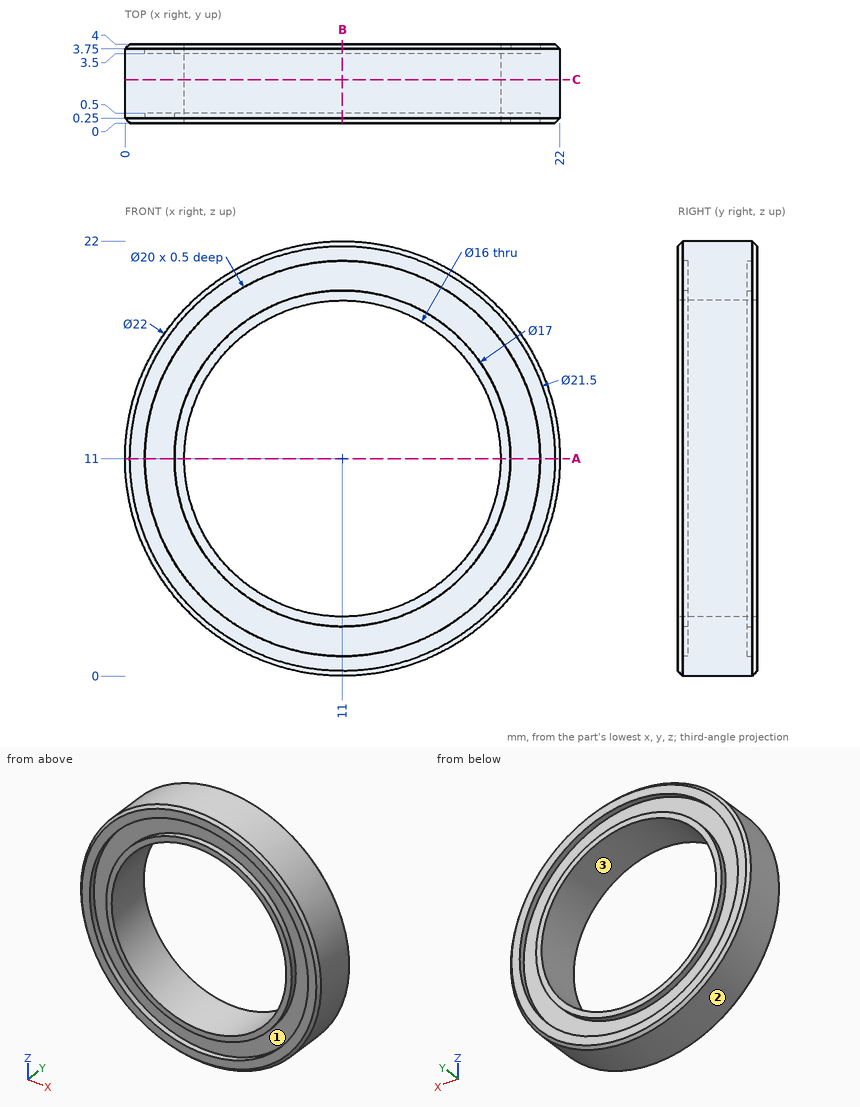
Print and shaded views of the part. All mm, measured from the part's lowest x, y and z. Give positions to 0.01 mm unless a question says otherwise; leave off trailing zeros. Write each loop counter-clockwise with the first axis right and the second up, starting at its lowest first coordinate (ties: lowest second). Pieces come first, ordered by that corner, then holes. Notation, with made-up numbers: (-26.5, 70.25) - (7.5, 70.25) arc R10 ccw to (7.5, 75.25) - close; hole circle Ø9 at (86, 47). An arc over 180 degrees is marked (long way). Put each result on its own line as item: value.
(1) Pull direction Z, two halves, no side cores. Call the marked faces 1, 2 and 3: released by +Z, released by -Z, zero draft, split by the parting line, or undercut.
Working result:
face 1: undercut
face 2: split by the parting line
face 3: undercut
(2) Drop flat-ended pins along their axis: pin 1 Ø5 at (x, z) = (7, 15) entering from -Y; pin 2 Ø1.5 at (y, z) = (3.5, 9.5) entering from -X. Give the stop position or say it passes through.
Working result:
pin 1: y = 0
pin 2: x = 0.03
(3) Saw through at C-C (y = 2.2). List the corners of the cut face in (x, z).
Working result:
outline: circle Ø22 at (11, 11); hole circle Ø16 at (11, 11)
(4) Wall check: L1, parallel to Z at x = 11, y = 3.8; L2, parallel to Y at x = 14.75, z = 19; L3, parallel to Z at x = 7.25, y = 2.8. Give the ranges that are in metal, low to high.
Working result:
L1: 0.05 to 1, 2.5 to 3, 19 to 19.5, 21 to 21.95
L2: 0.5 to 3.5
L3: 0.66 to 3.93, 18.07 to 21.34
(5) Saw through at A-A (z = 11). List the corners of the cut face in (x, y).
Working result:
outline: (0, 0.25) - (0.25, 0) - (1, 0) - (1, 0.5) - (2.5, 0.5) - (2.5, 0) - (3, 0) - (3, 4) - (2.5, 4) - (2.5, 3.5) - (1, 3.5) - (1, 4) - (0.25, 4) - (0, 3.75) - close; (19, 0) - (19.5, 0) - (19.5, 0.5) - (21, 0.5) - (21, 0) - (21.75, 0) - (22, 0.25) - (22, 3.75) - (21.75, 4) - (21, 4) - (21, 3.5) - (19.5, 3.5) - (19.5, 4) - (19, 4) - close
(6) Saw through at B-B (x = 11). List the corners of the cut face in (y, z), then the cut area to 3 significant figures.
Working result:
outline: (0, 0.25) - (0.25, 0) - (3.75, 0) - (4, 0.25) - (4, 1) - (3.5, 1) - (3.5, 2.5) - (4, 2.5) - (4, 3) - (0, 3) - (0, 2.5) - (0.5, 2.5) - (0.5, 1) - (0, 1) - close; (0, 19) - (4, 19) - (4, 19.5) - (3.5, 19.5) - (3.5, 21) - (4, 21) - (4, 21.75) - (3.75, 22) - (0.25, 22) - (0, 21.75) - (0, 21) - (0.5, 21) - (0.5, 19.5) - (0, 19.5) - close
area: 20.9 mm^2
